The model under review builds one solid part; all positions refer to its coordinate system, in mm. Face numbers are marked on the shaded views. A direction names the side the tool comes from. Coordinates: 2 decimals unless noted, no trailing zeros. Order: outer loops, then holes, each group sorted by start corner. A loop starts at its lowest first (then second) coordinate and runs counter-clockwise, first axis right, second up. Notation, with made-up numbers: (-27, -39.75) -> (20, -39.75) arc R34 cw to (20, -6.75) -> close; hole circle Ø4 at (21, 5). An arc over 180 degrees is marked (long way). Use one line per item in the form item = value. Start each with the question number.
(1) Take a section at B-B (y = 35.25). State the section outline as (x, z) points, then the cut area to 3 significant figures.
(2) Insertion check: pin 1 Ø11.5 at (x, y) = (0, 35.25) entering from -Z; pin 2 Ø6 at (x, z) = (-61, 11.5) entering from +Y; pin 3 Ø1.5 at (x, z) = (27.5, 22) entering from +Y. Each pin has a flat end and moves straight along its axis. Give the tip position at first contact, or say it passes through.
(3) Take a section at A-A (x = 0). State the section outline as (y, z) points.
(4) Take a section at C-C (z = -28). State the section outline as (x, y) points.
(5) For the marked faces 1 and 2, list the 3-axis set-ups (+Z, -Z, +X, -X, +Y, -Y) from which the entire face can be reached by the end or side of a thin tool; tool diameter is ignored.
(6) Wall thickness on line 1 along X through (y, z) = (18, 2); line 2 along X through (y, z) = (3, 0); line 3 along Y through (x, z) = (0, 63): over which ranges is each line inside the solid? List them lowest first.
(7) Mouldability with a two-part tool opening along X and no side actions: class the marked faces 3, 4 and 5 as +X half, -X half, draft (parallel to the pull), parting line (faces both ways), or undercut.
(8) Take a section at D-D (y = 17). State the section outline as (x, z) points.
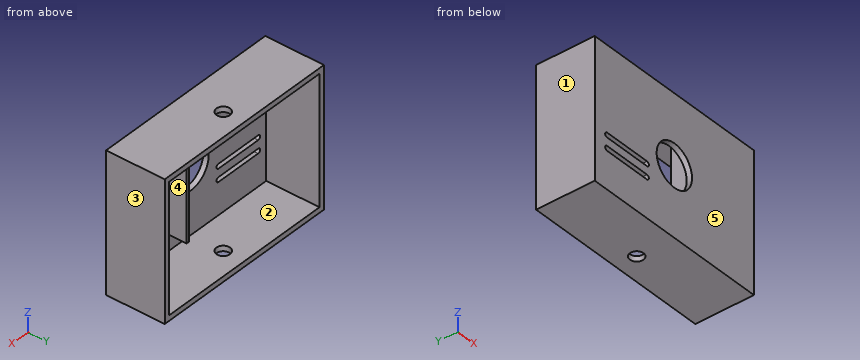
```python
from build123d import *

# Parameters (mm, degrees)
ESQUISSE1_W             = 180
ESQUISSE1_H             = 130
ESQUISSE1_W_2           = 170
ESQUISSE1_H_2           = 120
BOSS_EXTRU_2_DEPTH      = 55
ESQUISSE2_W             = 170
ESQUISSE2_H             = 120
BOSS_EXTRU_3_DEPTH      = 5
ESQUISSE3_R             = 20
ENL_V_MAT_EXTRU_1_DEPTH = 122.757956619
ENL_V_MAT_EXTRU_2_DEPTH = 122.757956619
ENL_V_MAT_EXTRU_3_REACH = 169.407
ESQUISSE5_R             = 6.35
ESQUISSE6_W             = 3
ESQUISSE6_H             = 101.6
BOSS_EXTRU_4_DEPTH      = 20


with BuildPart() as part:
    # Esquisse1 → Boss.-Extru.2 (new body)
    with BuildSketch(Plane(origin=(0, 0, 0), x_dir=(1, 0, 0), z_dir=(0, 1, 0))):
        Rectangle(ESQUISSE1_W, ESQUISSE1_H)
        Rectangle(ESQUISSE1_W_2, ESQUISSE1_H_2, mode=Mode.SUBTRACT)
    extrude(amount=BOSS_EXTRU_2_DEPTH)

    # Esquisse2 → Boss.-Extru.3 (add)
    with BuildSketch(Plane(origin=(0, 0, 0), x_dir=(1, 0, 0), z_dir=(0, 1, 0))):
        Rectangle(ESQUISSE2_W, ESQUISSE2_H)
    extrude(amount=BOSS_EXTRU_3_DEPTH)

    # Esquisse3 → Enlèv. mat.-Extru.1 (cut, through all)
    with BuildSketch(Plane(origin=(0, 5, 0), x_dir=(1, 0, 0), z_dir=(0, 1, 0))):
        with Locations(Location((0, 0, 0), (0, 0, 270))):
            Circle(ESQUISSE3_R)
    extrude(amount=-ENL_V_MAT_EXTRU_1_DEPTH, mode=Mode.SUBTRACT)

    # Esquisse4 → Enlèv. mat.-Extru.2 (cut, through all)
    with BuildSketch(Plane(origin=(0, 5, 0), x_dir=(1, 0, 0), z_dir=(0, 1, 0))):
        with BuildLine():
            Line((-76, 30.2), (-31, 30.2))
            ThreePointArc((-31, 30.2), (-28.8, 28), (-31, 25.8))
            Line((-31, 25.8), (-76, 25.8))
            ThreePointArc((-76, 25.8), (-78.2, 28), (-76, 30.2))
        make_face()
        with BuildLine():
            Line((-76, 18.2), (-31, 18.2))
            ThreePointArc((-31, 18.2), (-28.8, 16), (-31, 13.8))
            Line((-31, 13.8), (-76, 13.8))
            ThreePointArc((-76, 13.8), (-78.2, 16), (-76, 18.2))
        make_face()
    extrude(amount=-ENL_V_MAT_EXTRU_2_DEPTH, mode=Mode.SUBTRACT)

    # Enlèv. mat.-Extru.3: up to this face of the body (flat: up to its plane)
    enl_v_mat_extru_3_end = Plane(part.part.faces().sort_by_distance((0, 27.5, 65))[0])
    # Esquisse5 → Enlèv. mat.-Extru.3 (cut, up to the picked face)
    with BuildSketch(Plane(origin=(0, 0, -65), x_dir=(-1, 0, 0), z_dir=(0, 0, -1)), mode=Mode.PRIVATE) as enl_v_mat_extru_3_sk1:
        with Locations((0, 35.25)):
            Circle(ESQUISSE5_R)
    enl_v_mat_extru_3_tool1 = split(extrude(enl_v_mat_extru_3_sk1.sketch, amount=-ENL_V_MAT_EXTRU_3_REACH, mode=Mode.PRIVATE), bisect_by=enl_v_mat_extru_3_end, keep=Keep.BOTH, mode=Mode.PRIVATE)
    add(enl_v_mat_extru_3_tool1.solids().sort_by(Axis((0, 35.25, -65), (0, 0, 1)))[0], mode=Mode.SUBTRACT)

    # Esquisse6 → Boss.-Extru.4 (add)
    with BuildSketch(Plane(origin=(0, 5, 0), x_dir=(1, 0, 0), z_dir=(0, 1, 0))):
        with Locations((27.62, -9.2)):
            Rectangle(ESQUISSE6_W, ESQUISSE6_H)
    extrude(amount=BOSS_EXTRU_4_DEPTH)


solid = part.part
```
Findings:
q1.outline = (-90, -65) -> (-6.35, -65) -> (-6.35, -60) -> (-85, -60) -> (-85, 60) -> (-6.35, 60) -> (-6.35, 65) -> (-90, 65) -> close; (6.35, -65) -> (90, -65) -> (90, 65) -> (6.35, 65) -> (6.35, 60) -> (85, 60) -> (85, -60) -> (6.35, -60) -> close
q1.area = 2,870 mm²
q2.pin_1 = through
q2.pin_2 = 5
q2.pin_3 = 25
q3.outline = (0, -65) -> (28.9, -65) -> (28.9, -60) -> (5, -60) -> (5, -20) -> (0, -20) -> close; (0, 20) -> (5, 20) -> (5, 60) -> (28.9, 60) -> (28.9, 65) -> (0, 65) -> close; (41.6, -65) -> (55, -65) -> (55, -60) -> (41.6, -60) -> close; (41.6, 60) -> (55, 60) -> (55, 65) -> (41.6, 65) -> close
q4.outline = (-90, 0) -> (-78.2, 0) -> (-78.2, 5) -> (-85, 5) -> (-85, 55) -> (-90, 55) -> close; (-28.8, 0) -> (90, 0) -> (90, 55) -> (85, 55) -> (85, 5) -> (29.12, 5) -> (29.12, 25) -> (26.12, 25) -> (26.12, 5) -> (-28.8, 5) -> close
q5.face_1 = +Z, -Z, -X, +Y, -Y
q5.face_2 = +Y
q6.line_1 = -90 to -85, 26.12 to 29.12, 85 to 90
q6.line_2 = -90 to -20, 20 to 90
q6.line_3 = 0 to 28.9, 41.6 to 55
q7.face_3 = +X half
q7.face_4 = undercut
q7.face_5 = draft
q8.outline = (-90, -65) -> (90, -65) -> (90, 65) -> (-90, 65) -> close; hole (-85, -60) -> (85, -60) -> (85, 60) -> (29.12, 60) -> (29.12, -41.6) -> (26.12, -41.6) -> (26.12, 60) -> (-85, 60) -> close
